Model file for the job. Use its own axes, mm. Face numbers are marked on the shaded views. A direction names the side the tool comes from. Coordinates: 2 decimals unless noted, no trailing zeros. Order: outer loops, then holes, each group sorted by start corner. A loop starts at its lowest first (then second) coordinate and runs counter-clockwise, first axis right, second up. Notation, with made-up numbers: (-15, 71) -> (-2, 71) arc R10 ccw to (-2, 77) -> close; hole circle Ø7 at (-29, -26). An arc over 180 degrees is marked (long way). Write item = value, one per line. Start each with the question number.
Q1. Cut at C-C, the plane z = 180. List the corners of the cut face in (x, y), plus the area to 3 significant figures.
Q2. Flat gauge pins, fed straight in: pin 1 (5 mm diameter, centred on x = -2.5, z = 90.5, fed in from -Y); pin 2 (4 mm diameter, centred on y = 0.5, z = 111.5, fed in from -X); pin 3 (1.5 mm diameter, centred on y = -12, z = 53, fed in from +X); pin 4 (5 mm diameter, centred on x = 15, y = -8.5, fed in from -Z). Where does each tip first touch, or does it go through?
Q3. Cut at D-D, the plane y = 12. List the corners of the cut face in (x, z).
Q4. Cut at B-B, the plane y = 0. List the corners of the cut face in (x, z).
Q5. Cut at A-A, the plane x = 0. List the corners of the cut face in (y, z).
Q6. Wall check: line 1 (Z direction, x = 0, y = 8); line 2 (Z direction, x = 0.5, y = -18.5); line 3 (X direction, y = -1, z = 35). Give the ranges that are in metal, low to high. Write a range as from..to.
Q7. 3-axis set-ups, long thin cutter, end or side, ignore diameter. For the marked faces 1 and 2: which of +Z, -Z, +X, -X, +Y, -Y reach the whole face in a straight line?
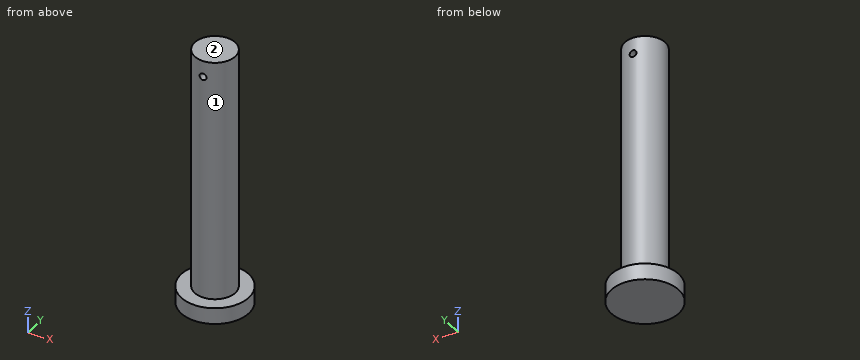
from build123d import *

# Parameters (mm, degrees)
SKETCH1_R               = 25
BOSS_EXTRUDE1_DEPTH     = 12
SKETCH2_R               = 15
BOSS_EXTRUDE2_DEPTH     = 180
CUT_EXTRUDE1_DEPTH      = 196.228071752
CUT_EXTRUDE1_DEPTH_BACK = 196.228071752
SKETCH3_R               = 2.5


with BuildPart() as part:
    # Sketch1 → Boss-Extrude1 (new body)
    with BuildSketch(Plane.XY):
        Circle(SKETCH1_R)
    extrude(amount=BOSS_EXTRUDE1_DEPTH)

    # Sketch2 → Boss-Extrude2 (add)
    with BuildSketch(Plane.XY.offset(12)):
        with Locations(Location((0, 0, 0), (0, 0, 180))):
            Circle(SKETCH2_R)
    extrude(amount=BOSS_EXTRUDE2_DEPTH)

    # Sketch3 → Cut-Extrude1 (cut, two sides: drawn at the far end of the back side and taken through both)
    with BuildSketch(Plane(origin=(0, 0, 0), x_dir=(1, 0, 0), z_dir=(0, 1, 0)).offset(-CUT_EXTRUDE1_DEPTH_BACK)):
        with Locations(Location((0, -180, 0), (0, 0, 270))):
            Circle(SKETCH3_R)
    extrude(amount=CUT_EXTRUDE1_DEPTH + CUT_EXTRUDE1_DEPTH_BACK, mode=Mode.SUBTRACT)


solid = part.part
Here are the results:
q1.outline = (-2.5, -14.79) -> (-2.5, 14.79) arc R15 ccw to start; (2.5, -14.79) arc R15 ccw to (2.5, 14.79) -> close
q1.area = 558 mm²
q2.pin_1 = -15
q2.pin_2 = -15
q2.pin_3 = 9.92
q2.pin_4 = 0
q3.outline = (-21.93, 0) -> (21.93, 0) -> (21.93, 12) -> (9, 12) -> (9, 192) -> (-9, 192) -> (-9, 12) -> (-21.93, 12) -> close; hole circle Ø5 at (0, 180)
q4.outline = (-25, 0) -> (25, 0) -> (25, 12) -> (15, 12) -> (15, 192) -> (-15, 192) -> (-15, 12) -> (-25, 12) -> close; hole circle Ø5 at (0, 180)
q5.outline = (-25, 0) -> (25, 0) -> (25, 12) -> (15, 12) -> (15, 177.5) -> (-15, 177.5) -> (-15, 12) -> (-25, 12) -> close; (-15, 182.5) -> (15, 182.5) -> (15, 192) -> (-15, 192) -> close
q6.line_1 = 0..177.5, 182.5..192
q6.line_2 = 0..12
q6.line_3 = -14.97..14.97
q7.face_1 = +Z
q7.face_2 = +Z, +X, -X, +Y, -Y
